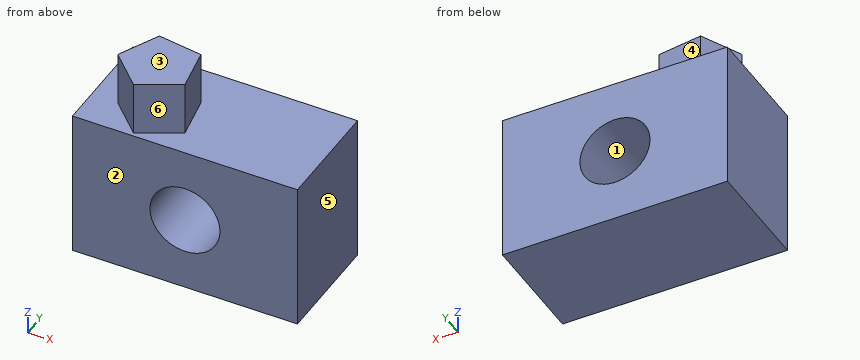
from build123d import *

# Parameters (mm, degrees)
F0_W     = 152.4
F0_H     = 101.6
F1_DEPTH = 76.2
F2_R     = 23.715347
F3_DEPTH = 76.201
F5_DEPTH = 36.57971


with BuildPart() as f1:
    # F0 (on Front) → F1 (new body)
    with BuildSketch(Plane.XZ):
        Rectangle(F0_W, F0_H)
    extrude(amount=F1_DEPTH)

    # F2 (on face) → F3 (cut, through all)
    with BuildSketch(Plane.XZ.offset(76.2)):
        Circle(F2_R)
    extrude(amount=-F3_DEPTH, mode=Mode.SUBTRACT)

    # F4 (on face) → F5 (join)
    with BuildSketch(Plane.XY.offset(50.8)):
        Polygon((-14.505152, -28.816074), (-44.9058, -24.522467), (-58.38358, -52.108403), (-36.312659, -73.451057), (-9.194299, -59.055606), align=None)
    extrude(amount=F5_DEPTH)


solid = f1.part
CAD build for the part. Positions are in the model's coordinates, mm. Face numbers are marked on the shaded views. A direction names the side the tool comes from. Give positions to 0.01 mm unless a question says otherwise; leave off trailing zeros. Loops run counter-clockwise (first coordinate to the right, second up) from the corner with the lowest first, then second, coordinate; pieces in that order, holes last. Notation, with made-up numbers: M 6.5,-29 L 13.5,-29 A25 ccw 13.5,5 Z; hole C -19,-26 d6. An arc over 180 degrees is marked long. Answer in a Markdown table with one row per item. Add a question column.
Item 1: Drop flat-ended pins along their axis: P1, Ø3, axis at x = -32.5, z = 62.5, coming from the -Y side; P2, Ø2, axis at y = -60, z = 73, coming from the -X side. Give the stop position or say it passes through.
Item 2: Mould opens along Z. For the marked faces 1, 2 and 3 say: +Z half, -Z half, draft (parallel to the pull), parting line (faces both ways), or undercut.
Item 3: Band-saw the part on B-B on z = 0. Give the cut face in (x, y).
Item 4: Band-saw the part on C-C on y = -21. Give the cut face in (x, z).
Item 5: Probe probe 1 along Z at (x, y) = (0, -45); probe 2 along Z at (x, y) = (33.5, -43.5); probe 3 along Z at (x, y) = (-21, -50). List the from-to ranges inside material, lowest first.
Item 6: Band-saw the part on D-D on z = 57.5. Give the cut face in (x, y).
Item 7: Tool access for the marked faces 4, 5 and 6: list every direction of +Z, -Z, +X, -X, +Y, -Y with a clear straight run to the whole face (end or side of a thin tool).
Item 8: Band-saw the part on A-A on x = 0. Give the cut face in (y, z).
Reply:
| question | item | result |
|---|---|---|
| 1 | P1 | stops at y = -72.22 |
| 1 | P2 | stops at x = -51.26 |
| 2 | face 1 | undercut |
| 2 | face 2 | draft |
| 2 | face 3 | +Z half |
| 3 | outline | M -76.2,-76.2 L -23.72,-76.2 L -23.72,0 L -76.2,0 Z; M 23.72,-76.2 L 76.2,-76.2 L 76.2,0 L 23.72,0 Z |
| 4 | outline | M -76.2,-50.8 L 76.2,-50.8 L 76.2,50.8 L -76.2,50.8 Z; hole C 0,0 d47.43 |
| 5 | probe 1 | z = -50.8 to -23.72, 23.72 to 50.8 |
| 5 | probe 2 | z = -50.8 to 50.8 |
| 5 | probe 3 | z = -50.8 to -11.02, 11.02 to 87.38 |
| 6 | outline | M -58.38,-52.11 L -36.31,-73.45 L -9.19,-59.06 L -14.51,-28.82 L -44.91,-24.52 Z |
| 7 | face 4 | +Z, +X, +Y |
| 7 | face 5 | +Z, -Z, +X, +Y, -Y |
| 7 | face 6 | +Z, +X, -Y |
| 8 | outline | M -76.2,-50.8 L 0,-50.8 L 0,-23.72 L -76.2,-23.72 Z; M -76.2,23.72 L 0,23.72 L 0,50.8 L -76.2,50.8 Z |
